from build123d import *

# Parameters (mm, degrees)
F0_R      = 33.5
F0_R_2    = 32
F1_DEPTH  = 30
F0_R_3    = 30
F0_R_4    = 28.8
F2_R      = 33.5
F3_DEPTH  = 2
F5_DEPTH  = 12
F6_SIZE   = 11.9999
F6_2_SIZE = 11.9999
F6_3_SIZE = 11.9999
F8_R      = 6.5
F9_DEPTH  = 25


# Not quite as in the source:
# - a fillet or chamfer is up to 0.001 mm smaller than in the source, because OpenCascade refuses the exact size


with BuildPart() as f1:
    # F0 (on Top) → F1 (new body)
    with BuildSketch(Plane.XY):
        Circle(F0_R)
        Circle(F0_R_2, mode=Mode.SUBTRACT)
    extrude(amount=F1_DEPTH)


with BuildPart() as f1b:
    # F0 (on Top) → F1, piece 2 (new body)
    with BuildSketch(Plane.XY):
        Circle(F0_R_3)
        Circle(F0_R_4, mode=Mode.SUBTRACT)
    extrude(amount=F1_DEPTH)


with BuildPart() as f3:
    # F2 (on face) → F3 (new body)
    with BuildSketch(Plane(origin=(0, 0, 0), x_dir=(1, 0, 0), z_dir=(0, 0, -1))):
        Circle(F2_R)
    extrude(amount=F3_DEPTH)


with BuildPart() as f5:
    # F4 (on face) → F5 (new body)
    with BuildSketch(Plane.XY):
        with BuildLine():
            Line((9.993418715, 25.1754931604), (10.5667748746, 26.7914775395))
            ThreePointArc((10.5667748746, 26.7914775395), (10.0999818657, 26.9709170462), (9.630143492, 27.1422242332))
            Line((9.630143492, 27.1422242332), (9.993418715, 25.1754931604))
        make_face()
        with BuildLine():
            Line((8.1085420321, 25.8442531252), (9.630143492, 27.1422242332))
            ThreePointArc((9.630143492, 27.1422242332), (9.15740142, 27.3053474476), (8.6818981918, 27.4602375042))
            Line((8.6818981918, 27.4602375042), (8.1085420321, 25.8442531252))
        make_face()
        Polygon((9.993418715, 25.1754931604), (9.630143492, 27.1422242332), (5.6175837037, 15.832964136), (6.5600220451, 15.4985841536), align=None)
        Polygon((5.6175837037, 15.832964136), (9.630143492, 27.1422242332), (8.1085420321, 25.8442531252), (4.6751453622, 16.1673441184), align=None)
    extrude(amount=F5_DEPTH)

    # F6#2 (size 12 in the source; OpenCascade refuses exactly that, so slightly less here)
    f6_2_edges = [f5.edges().sort_by_distance(p)[0] for p in [
        (5.617584, 15.832964, 12),
    ]]
    chamfer(f6_2_edges, length=F6_2_SIZE)


with BuildPart() as f5b:
    # F4 (on face) → F5, piece 2 (new body)
    with BuildSketch(Plane.XY):
        with BuildLine():
            Line((-26.769701888, -3.9079218685), (-28.488352252, -4.2253740625))
            ThreePointArc((-28.488352252, -4.2253740625), (-28.4090912902, -4.7290096283), (-28.3209274471, -5.2311632104))
            Line((-28.3209274471, -5.2311632104), (-26.769701888, -3.9079218685))
        make_face()
        with BuildLine():
            ThreePointArc((-28.3209274471, -5.2311632104), (-28.2277588918, -5.7125850495), (-28.1264073572, -6.1923508604))
            Line((-28.1264073572, -6.1923508604), (-26.4727474785, -5.8869030696))
            Line((-26.4727474785, -5.8869030696), (-28.3209274471, -5.2311632104))
        make_face()
        Polygon((-16.7057304605, -2.0490040353), (-26.769701888, -3.9079218685), (-28.3209274471, -5.2311632104), (-16.5205565416, -3.0515147414), (-16.5240928491, -3.0323695717), align=None)
        Polygon((-28.3209274471, -5.2311632104), (-26.4727474785, -5.8869030696), (-16.3424552376, -4.0157351081), (-16.5205565416, -3.0515147414), align=None)
    extrude(amount=F5_DEPTH)

    # F6 (size 12 in the source; OpenCascade refuses exactly that, so slightly less here)
    f6_edges = [f5b.edges().sort_by_distance(p)[0] for p in [
        (-16.524093, -3.03237, 12),
    ]]
    chamfer(f6_edges, length=F6_SIZE)


with BuildPart() as f5c:
    # F4 (on face) → F5, piece 3 (new body)
    with BuildSketch(Plane.XY):
        with BuildLine():
            ThreePointArc((17.9187127168, -22.5468342472), (18.3075083925, -22.2322993966), (18.6907839551, -21.9110610228))
            Line((18.6907839551, -21.9110610228), (16.8059072723, -21.242301058))
            Line((16.8059072723, -21.242301058), (17.9187127168, -22.5468342472))
        make_face()
        with BuildLine():
            ThreePointArc((18.6907839551, -21.9110610228), (19.0684238388, -21.5832159862), (19.4403141767, -21.2488631392))
            Line((19.4403141767, -21.2488631392), (18.3275087322, -19.94432995))
            Line((18.3275087322, -19.94432995), (18.6907839551, -21.9110610228))
        make_face()
        Polygon((10.9029573072, -12.7814522633), (18.6907839551, -21.9110610228), (18.3275087322, -19.94432995), (11.6637580371, -12.1324667093), align=None)
        Polygon((16.8059072723, -21.242301058), (18.6907839551, -21.9110610228), (10.9029573072, -12.7814522633), (10.1421565772, -13.4304378173), align=None)
    extrude(amount=F5_DEPTH)

    # F6#3 (size 12 in the source; OpenCascade refuses exactly that, so slightly less here)
    f6_3_edges = [f5c.edges().sort_by_distance(p)[0] for p in [
        (10.902957, -12.781452, 12),
    ]]
    chamfer(f6_3_edges, length=F6_3_SIZE)


with BuildPart() as f5_1:
    add(f5.part)

    # F7: union F1b, F1, F3, F5b, F5c
    add(f1b.part)
    add(f1.part)
    add(f3.part)
    add(f5b.part)
    add(f5c.part)

    # F8 (on face) → F9 (cut)
    with BuildSketch(Plane.XY):
        Circle(F8_R)
    extrude(amount=-F9_DEPTH, mode=Mode.SUBTRACT)


solid = f5_1.part
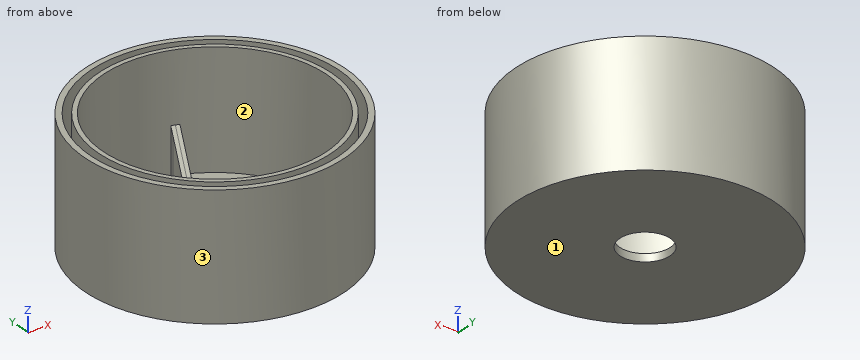
The listing builds one solid part. Answer for the finished solid, in the listing's coordinates (mm). Face numbers are marked on the shaded views. Give positions to 0.01 mm unless a question says otherwise; leave off trailing zeros. Order: outer loops, then holes, each group sorted by start corner. A loop starts at its lowest first (then second) coordinate and runs counter-clockwise, first axis right, second up. Notation, with made-up numbers: (0.25, 35.5) -> (59.25, 35.5) arc R11 ccw to (59.25, 52.5) -> close; hole circle Ø5 at (40.5, 32.25). An arc over 180 degrees is marked (long way). Put each result on its own line as item: value.
Item 1: For a pull along X with two mould halves and no side action, classify the marked faces 1, 2 and 3 as released by +X, released by -X, zero draft, split by the parting line, or undercut.
Established:
face 1: zero draft
face 2: undercut
face 3: split by the parting line
Item 2: A cutting plane is placed at C-C on z = 6.5. Give the vertices of the cut face in (x, y), plus the area to 3 significant figures.
Established:
outline: circle Ø67 at (0, 0); circle Ø60 at (0, 0); hole circle Ø64 at (0, 0); hole (-28.49, -4.23) -> (-23.1, -3.23) -> (-22.73, -5.2) -> (-28.13, -6.19) arc R28.8 ccw to (17.92, -22.55) -> (14.36, -18.38) -> (15.88, -17.08) -> (19.44, -21.25) arc R28.8 ccw to (10.57, 26.79) -> (8.73, 21.62) -> (6.85, 22.29) -> (8.68, 27.46) arc R28.8 ccw to start
area: 563 mm^2
Item 3: A cutting plane is placed at A-A on x = 0. Give the vertices of the cut face in (y, z).
Established:
outline: (-33.5, -2) -> (-6.5, -2) -> (-6.5, 0) -> (-28.8, 0) -> (-28.8, 30) -> (-30, 30) -> (-30, 0) -> (-32, 0) -> (-32, 30) -> (-33.5, 30) -> close; (6.5, -2) -> (33.5, -2) -> (33.5, 30) -> (32, 30) -> (32, 0) -> (30, 0) -> (30, 30) -> (28.8, 30) -> (28.8, 0) -> (6.5, 0) -> close
Item 4: Given P1, Ø1, axis at x = -17.5, z = 9.5, coming from the +Y side; P2, Ø12, axis at x = -26, z = 26, coming from the +Y side; P3, Ø6, axis at x = -0.5, y = 6.5, coming from the +Z side, each flat-ended and moving along its own axis, determine where each tip first touches the part or whether it passes through.
Established:
P1: stops at y = 28.87
P2: stops at y = 26.87
P3: stops at z = 0
Item 5: Straight lines are drawn through the part: line 1 (Y direction, x = 0, z = 23); line 2 (X direction, y = 22, z = 15); line 3 (X direction, y = -25, z = 1). For each, find the intervals that lie inside material, in ascending order.
Established:
line 1: y = -33.5 to -32, -30 to -28.8, 28.8 to 30, 32 to 33.5
line 2: x = -25.26 to -23.24, -20.4 to -18.59, 18.59 to 20.4, 23.24 to 25.26
line 3: x = -22.3 to -19.97, -16.58 to -14.3, 14.3 to 16.58, 19.97 to 22.3
Item 6: A cutting plane is placed at D-D on z = 19. Give the vertices of the cut face in (x, y).
Established:
outline: circle Ø67 at (0, 0); circle Ø60 at (0, 0); hole circle Ø64 at (0, 0); hole circle Ø57.6 at (0, 0)
